```python
from build123d import *

# Parameters (mm, degrees)
BOSS_EXTRUDE1_DEPTH = 1.5
SKETCH2_R           = 1.55
CUT_EXTRUDE1_DEPTH  = 54.49517282


with BuildPart() as part:
    # Sketch1 → Boss-Extrude1 (new body)
    with BuildSketch(Plane.XY):
        with BuildLine():
            Line((-10.351321581, 8), (-10.351321581, 45.1))
            Line((-10.351321581, 45.1), (-9.925677234, 45.1))
            Line((-9.925677234, 45.1), (-9.786312195, 45.1))
            ThreePointArc((-9.786312195, 45.1), (-4.668121471, 46.363259082), (-0.725494549, 49.862886598))
            ThreePointArc((-0.725494549, 49.862886598), (2.198678419, 51.4), (5.122851386, 49.862886598))
            ThreePointArc((5.122851386, 49.862886598), (9.065478308, 46.363259082), (14.183669032, 45.1))
            Line((14.183669032, 45.1), (14.323034072, 45.1))
            Line((14.323034072, 45.1), (14.748678419, 45.1))
            Line((14.748678419, 45.1), (14.748678419, 8))
            Line((14.748678419, 8), (14.183669032, 8))
            ThreePointArc((14.183669032, 8), (9.065478308, 6.736740918), (5.122851386, 3.237113402))
            ThreePointArc((5.122851386, 3.237113402), (2.198678419, 1.7), (-0.725494549, 3.237113402))
            ThreePointArc((-0.725494549, 3.237113402), (-4.668121471, 6.736740918), (-9.786312195, 8))
            Line((-9.786312195, 8), (-10.351321581, 8))
        make_face()
    extrude(amount=BOSS_EXTRUDE1_DEPTH)

    # Sketch2 → Cut-Extrude1 (cut, through all)
    with BuildSketch(Plane.XY.offset(1.5)):
        with Locations((2.198678419, 47.85)):
            Circle(SKETCH2_R)
        with Locations((2.198678419, 5.25)):
            Circle(SKETCH2_R)
    extrude(amount=-CUT_EXTRUDE1_DEPTH, mode=Mode.SUBTRACT)


solid = part.part
```
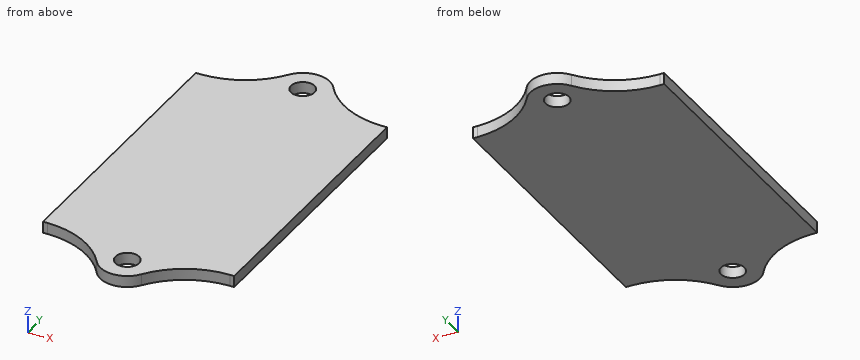
Could you check a few things on this model? Use its own coordinates, in mm. Coordinates: 2 decimals unless noted, no trailing zeros. Write each loop counter-clockwise with the first axis right and the second up, starting at its lowest first coordinate (ties: lowest second). Pieces come first, ordered by that corner, then holes. Notation, with made-up numbers: (61, -22.5) - (83, -22.5) arc R22 cw to (83, 7.5) - close; hole circle Ø11 at (12.5, 24). An arc over 180 degrees is marked (long way). Use a Markdown table: item, result.
Q1. Imagine slicing it at D-D (x = 9). List the corners of the cut face in (y, z) for me.
Geometry check:
| item | result |
|---|---|
| outline | (6.7, 0) - (46.4, 0) - (46.4, 1.5) - (6.7, 1.5) - close |
Q2. Please list where these lines run through material, in increasing order: L1, parallel to Y at x = 1, z = 1.15; L2, parallel to Y at x = -0.5, z = 0.7; L3, parallel to Y at x = 11.25, z = 0.2.
Geometry check:
| item | result |
|---|---|
| L1 | y = 1.91 to 4.27, 6.23 to 46.87, 48.83 to 51.19 |
| L2 | y = 2.94 to 50.16 |
| L3 | y = 7.6 to 45.5 |
Q3. I'm going to push a flat-ended pin straight in: pin 1 Ø0.6 at (x, z) = (-10, 1) entering from -Y. Where does the tip first touch, or does it pass through?
Geometry check:
| item | result |
|---|---|
| pin 1 | stops at y = 8 |
Q4. Imagine slicing it at B-B (y = 47.85). List the corners of the cut face in (x, z) for me, and give its area (3 significant figures).
Geometry check:
| item | result |
|---|---|
| outline | (-2.51, 0) - (0.65, 0) - (0.65, 1.5) - (-2.51, 1.5) - close; (3.75, 0) - (6.91, 0) - (6.91, 1.5) - (3.75, 1.5) - close |
| area | 9.48 mm2 |
Q5. Imagine slicing it at A-A (z = 0.4). List the corners of the cut face in (x, y) for me, and give its area (3 significant figures).
Geometry check:
| item | result |
|---|---|
| outline | (-10.35, 8) - (-9.79, 8) arc R11 cw to (-0.73, 3.24) arc R3.55 ccw to (5.12, 3.24) arc R11 cw to (14.18, 8) - (14.75, 8) - (14.75, 45.1) - (14.18, 45.1) arc R11 cw to (5.12, 49.86) arc R3.55 ccw to (-0.73, 49.86) arc R11 cw to (-9.79, 45.1) - (-10.35, 45.1) - close; hole circle Ø3.1 at (2.2, 5.25); hole circle Ø3.1 at (2.2, 47.85) |
| area | 1,040 mm2 |
Q6. Imagine slicing it at C-C (x = -1.5). List the corners of the cut face in (y, z) for me, and give its area (3 significant figures).
Geometry check:
| item | result |
|---|---|
| outline | (4.23, 0) - (48.87, 0) - (48.87, 1.5) - (4.23, 1.5) - close |
| area | 66.9 mm2 |
